```python
from build123d import *

# Parameters (mm, degrees)
F1_DEPTH = 20
F2_DEPTH = 5
F3_DEPTH = 4
F4_DEPTH = 15
F5_R     = 0.8
F6_DEPTH = 8.5841977808


# Not quite as in the source:
# - a feature names something its author has since deleted; it is built from what else it names


with BuildPart() as f1:
    # F0 (on Front) → F1 (new body)
    with BuildSketch(Plane.XZ):
        with BuildLine():
            ThreePointArc((15.7162336455, 3), (12.3288280059, -10.1980390272), (0, -16))
            Line((0, -16), (0, -20))
            ThreePointArc((0, -20), (7.8433854689, -18.397861408), (14.4301518825, -13.8481304387))
            ThreePointArc((14.4301518825, -13.8481304387), (17.9256749339, -8.8696210836), (19.762883185, -3.0705778311))
            ThreePointArc((19.762883185, -3.0705778311), (19.9970282657, 0.3447615687), (19.6452920569, 3.75))
            Line((19.6452920569, 3.75), (15.7162336455, 3))
        make_face()
    extrude(amount=F1_DEPTH)

    # F1_face (on face) → F2 (join)
    with BuildSketch(Plane(origin=(12.1989359317, 0, -10.0905961752), x_dir=(1, 0, 0), z_dir=(0, 1, 0))):
        with BuildLine():
            Line((3.5172977138, -13.0905961752), (7.4463561252, -13.8405961752))
            ThreePointArc((7.4463561252, -13.8405961752), (3.2120990757, 2.6569526088), (-12.1989359317, 9.9094038248))
            Line((-12.1989359317, 9.9094038248), (-12.1989359317, 5.9094038248))
            ThreePointArc((-12.1989359317, 5.9094038248), (0.1298920742, 0.107442852), (3.5172977138, -13.0905961752))
        make_face()
    extrude(amount=F2_DEPTH)

    # F0 (on Front) → F3 (join)
    with BuildSketch(Plane.XZ):
        with BuildLine():
            ThreePointArc((15.7162336455, 3), (12.3288280059, -10.1980390272), (0, -16))
            Line((0, -16), (0, -20))
            ThreePointArc((0, -20), (7.8433854689, -18.397861408), (14.4301518825, -13.8481304387))
            ThreePointArc((14.4301518825, -13.8481304387), (17.9256749339, -8.8696210836), (19.762883185, -3.0705778311))
            ThreePointArc((19.762883185, -3.0705778311), (19.9970282657, 0.3447615687), (19.6452920569, 3.75))
            Line((19.6452920569, 3.75), (15.7162336455, 3))
        make_face()
        with BuildLine():
            Line((21.3768143102, 4.080522368), (19.6452920569, 3.75))
            ThreePointArc((19.6452920569, 3.75), (19.9970282657, 0.3447615687), (19.762883185, -3.0705778311))
            Line((19.762883185, -3.0705778311), (22, -4.3621778265))
            Line((22, -4.3621778265), (25.5, 1.7))
            Line((25.5, 1.7), (21.3768143102, 4.080522368))
        make_face()
        with BuildLine():
            ThreePointArc((19.762883185, -3.0705778311), (17.9256749339, -8.8696210836), (14.4301518825, -13.8481304387))
            Line((14.4301518825, -13.8481304387), (16, -14.7544826719))
            Line((16, -14.7544826719), (22, -4.3621778265))
            Line((22, -4.3621778265), (19.762883185, -3.0705778311))
        make_face()
    extrude(amount=F3_DEPTH)

    # F0 (on Front) → F4 (join)
    with BuildSketch(Plane.XZ):
        with BuildLine():
            Line((21.3768143102, 4.080522368), (19.6452920569, 3.75))
            ThreePointArc((19.6452920569, 3.75), (19.9970282657, 0.3447615687), (19.762883185, -3.0705778311))
            Line((19.762883185, -3.0705778311), (22, -4.3621778265))
            Line((22, -4.3621778265), (25.5, 1.7))
            Line((25.5, 1.7), (21.3768143102, 4.080522368))
        make_face()
    extrude(amount=F4_DEPTH)

    # F5 (on face) → F6 (cut, through all)
    with BuildSketch(Plane(origin=(18.3888784068, 0, -10.6168238983), x_dir=(0, 1, 0), z_dir=(0.8660254038, 0, -0.5))):
        with Locations((-12.5, 11.7222431864)):
            Circle(F5_R)
        with Locations((-2.5, 11.7222431864)):
            Circle(F5_R)
    extrude(amount=-F6_DEPTH, mode=Mode.SUBTRACT)

    # F7: F1 across plane


with BuildPart() as f1_1:
    add(f1.part)
    add(f1.part.mirror(Plane.YZ))


solid = f1_1.part
```
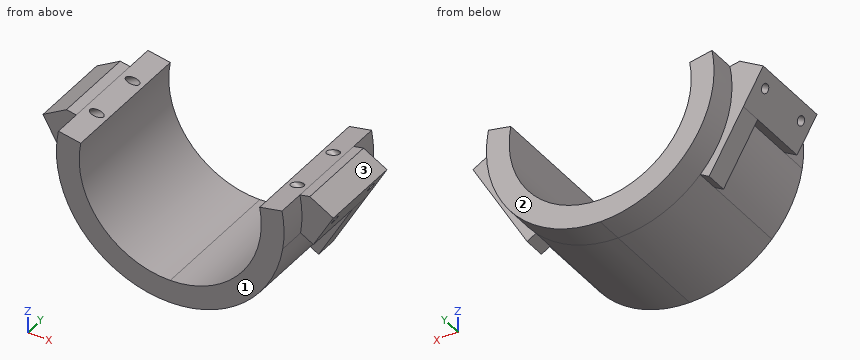
Geometry: final body of the model. Coordinates: model frame, mm. Face numbers are marked on the shaded views. Round coordinates to 2 decimals unless told otherwise and drop trailing zeros. Order: outer loops, then holes, each group sorted by start corner. A loop starts at its lowest first (then second) coordinate and runs counter-clockwise, first axis right, second up. Notation, with made-up numbers: (47, 53.25) - (82, 53.25) arc R13 ccw to (82, 65.25) - close; hole circle Ø5 at (-24, 20). An arc over 180 degrees is marked (long way). Write item = value, one per line. Start each with the question number.
Q1. Cut plane C-C on x = -11.5. Return the cut outline in (y, z).
Q2. Pull-direction query (Y, two-part tool) for the marked faces 1, 2 and 3; classes: +Y half, -Y half, draft (parallel to the pull), parting line (faces both ways), or undercut.
Q3. Ray query, line 1 (Y direction, x = -20.5, z = -6.5); line 2 (X direction, y = -0.75, z = -10) (3 decimals); line 3 (X direction, y = -16.5, z = -13.25). Return the intervals inside material, ascending. Write a range as from..to.
Q4. Cut plane B-B on z = -9. Return the cut outline in (x, y).
Q5. Cut plane A-A on y = -14. Return the cut outline in (x, z).
Q6. Cut plane D-D on z = 0.75. Give the number of separate pieces and of enclosed holes in the cut face, and give its area (3 significant figures).
Q7. Pin query (flat end, axial travel): pin 1 (4.5 mm diameter, centred on x = -23.5, z = 0.5, fed in from -Y); pin 2 (3 mm diameter, centred on y = -5.5, z = 0, fed in from -X); pin 3 (6 mm diameter, centred on y = -13.5, z = -16.5, fed in from +X). Return the tip coordinate at first contact, or that it passes through.
Outcome:
q1.outline = (-20, -16.36) - (5, -16.36) - (5, -11.12) - (-20, -11.12) - close
q2.face_1 = -Y half
q2.face_2 = +Y half
q2.face_3 = draft
q3.line_1 = -4..0
q3.line_2 = -18.745..-12.49, 12.49..18.745
q3.line_3 = -14.98..-8.97, 8.97..14.98
q4.outline = (-19.32, -4) - (-17.86, -4) - (-17.86, -20) - (-13.23, -20) - (-13.23, 5) - (-17.86, 5) - (-17.86, 0) - (-19.32, 0) - close; (13.23, -20) - (17.86, -20) - (17.86, -4) - (19.32, -4) - (19.32, 0) - (17.86, 0) - (17.86, 5) - (13.23, 5) - close
q5.outline = (-25.5, 1.7) - (-22, -4.36) - (-19.76, -3.07) arc R20 ccw to (19.76, -3.07) - (22, -4.36) - (25.5, 1.7) - (21.38, 4.08) - (15.72, 3) arc R16 cw (long way) to (-15.72, 3) - (-21.38, 4.08) - close
q6.separate_pieces = 2
q6.enclosed_holes = 4
q6.area = 333 mm^2
q7.pin_1 = -15
q7.pin_2 = -25.38
q7.pin_3 = 14.76
